Check sheet for the modelled part. Datum: model origin and axes. Units: mm. Face numbers are marked on the shaded views. Round coordinates to 2 decimals unless told otherwise and drop trailing zeros. Write each loop counter-clockwise with the first axis right and the second up, starting at its lowest first coordinate (ties: lowest second). Pieces come first, ordered by that corner, then holes. Notation, with made-up numbers: (-20, 21) -> (14, 21) arc R16 cw to (14, 27) -> close; hole circle Ø11 at (-5, 44.25). An arc over 180 degrees is marked (long way). Write item = value, one per line.
Autodesk Inventor part; units mm, degrees
ref_plane "YZ Plane" through (0, 0, 0) normal (1, 0, 0) x (0, 1, 0)
ref_plane "XZ Plane" through (0, 0, 0) normal (0, 1, 0) x (-1, 0, 0)
ref_plane "XY Plane" through (0, 0, 0) normal (0, 0, 1) x (1, 0, 0)
sketch "Skizze1" plane through (0, 0, 0) normal (0, 0, 1) x (1, 0, 0)
  circle A0 centre (0, 0) radius 34.775
  dimension "d0" = 69.55
extrude "Extrusion1" add sketch "Skizze1" along normal blind 5
sketch "Skizze2" plane through (0, 0, 5) normal (0, 0, 1) x (1, 0, 0)
  circle A0 centre (0, 0) radius 32.54
  dimension "d3" = 65.08
extrude "Extrusion2" cut sketch "Skizze2" against normal blind 3
sketch "Skizze3" plane through (0, 0, 0) normal (0, 0, -1) x (-1, 0, 0)
  circle A0 centre (0, 0) radius 6.21
  dimension "d6" = 12.42
extrude "Extrusion3" cut sketch "Skizze3" against normal through all
sketch "Skizze4" plane through (0, 0, 5) normal (0, 0, 1) x (1, 0, 0)
  line L0 (-8, -42.775) -> (8, -42.775)
  line L1 (8, -42.775) -> (8, -26.775)
  line L2 (8, -26.775) -> (-8, -26.775)
  line L3 (-8, -26.775) -> (-8, -42.775)
  circle A0 centre (0, 0) radius 34.775
  line L4 (-8, -42.775) -> (8, -26.775) construction
  line L5 (8, -42.775) -> (-8, -26.775) construction
  point P0 (0, -34.775)
  dimension "d9" = 16
  dimension "d10" = 16
extrude "Extrusion4" cut sketch "Skizze4" against normal up to surface (3 mm away) contours L3 A0 L1 L0 | L3 L2 L1 A0 picked at (0.896, -29.407)
properties part number "2024_08_28_Holder_disk_GL14"
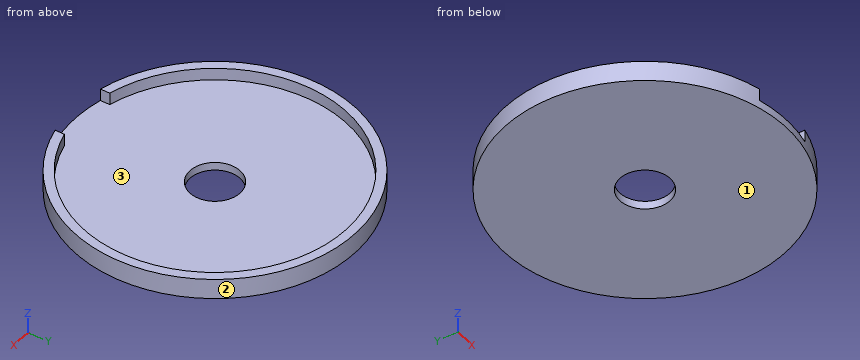
(1) Go/stop test with flat-tipped pins: P1, Ø2, axis at x = 4, z = 2, coming from the +Y side; P2, Ø1, axis at y = -25, z = 2, coming from the +X side; P3, Ø11, axis at x = 0, y = 0, coming from the -Z side; P4, Ø2, axis at x = 2, z = 1, coming from the -Y side. Record where each tip stops, or that it passes through.
Worked answers:
P1 = 34.65
P2 = 24.68
P3 = through
P4 = -34.76
(2) Sectioned sample at A-A on y = 0. Enter the section's corners in (x, z) (3 decimals).
Worked answers:
outline = (-34.775, 0) -> (-6.21, 0) -> (-6.21, 2) -> (-32.54, 2) -> (-32.54, 5) -> (-34.775, 5) -> close; (6.21, 0) -> (34.775, 0) -> (34.775, 5) -> (32.54, 5) -> (32.54, 2) -> (6.21, 2) -> close
(3) Material ranges on L1, parallel to Z at x = -16, y = -14; L2, parallel to Y at x = 0, z = 0.6 (3 decimals); L3, parallel to Y at x = -15, z = 4.8, recorded low to high. Write a range as [from, to].
Worked answers:
L1 = [0, 2]
L2 = [-34.775, -6.21], [6.21, 34.775]
L3 = [-31.37, -28.88], [28.88, 31.37]
(4) Sectioned sample at C-C on x = -16. Enter the section's corners in (y, z).
Worked answers:
outline = (-30.88, 0) -> (30.88, 0) -> (30.88, 5) -> (28.33, 5) -> (28.33, 2) -> (-28.33, 2) -> (-28.33, 5) -> (-30.88, 5) -> close
(5) Release check for a two-part mould opening along X. For the marked faces 1, 2 and 3 record: pulls with the +X half, pulls with the -X half, needs draft (parallel to the pull), parting line crosses it, or undercut.
Worked answers:
face_1 = needs draft
face_2 = parting line crosses it
face_3 = undercut
(6) Sectioned sample at B-B on x = 0. Enter the section's corners in (y, z) (3 decimals), then the cut area to 3 significant figures.
Worked answers:
outline = (-34.775, 0) -> (-6.21, 0) -> (-6.21, 2) -> (-34.775, 2) -> close; (6.21, 0) -> (34.775, 0) -> (34.775, 5) -> (32.54, 5) -> (32.54, 2) -> (6.21, 2) -> close
area = 121 mm²
